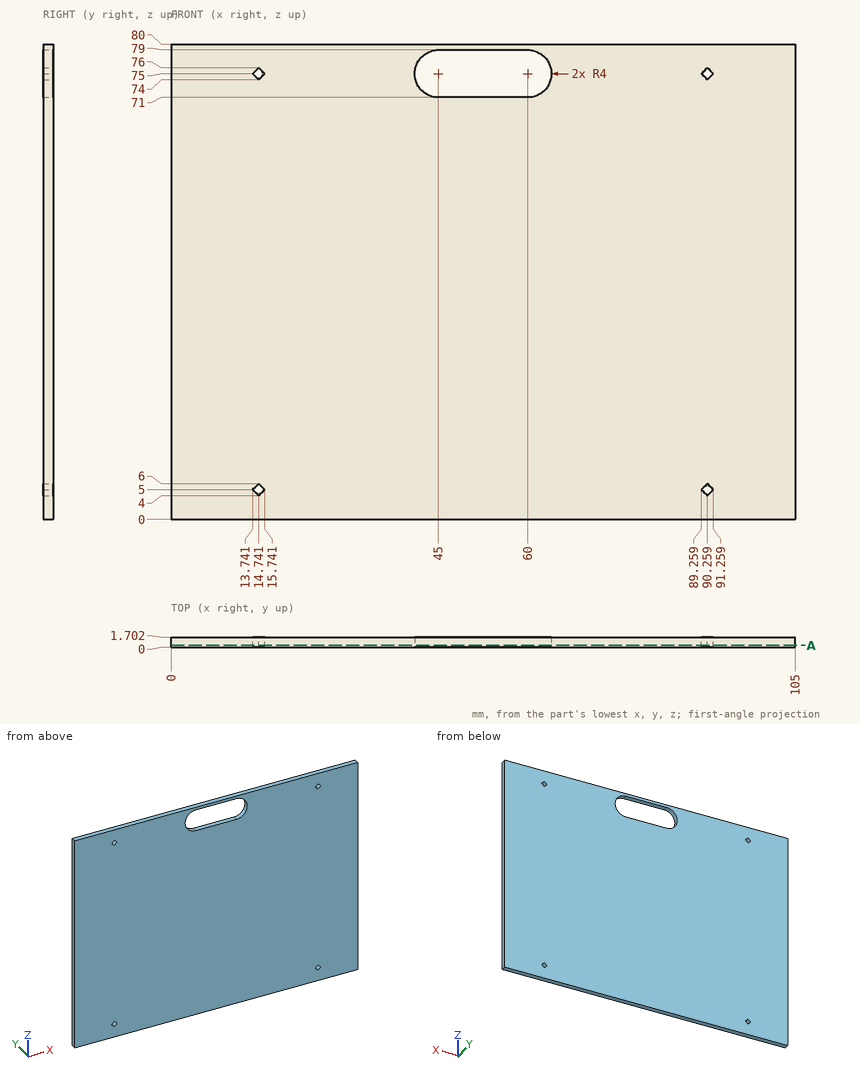
For this review, use the dimensioned drawing (mm, ordinates from the lowest corner) and the shaded views. Coordinates: 2 decimals unless noted, no trailing zeros. Loops run counter-clockwise (first coordinate to the right, second up) from the corner with the lowest first, then second, coordinate; pieces in that order, holes last. Notation, with made-up numbers: (72, 2) -> (100, 2) arc R27 ccw to (100, 26) -> close; hole circle Ø10 at (-17.75, 1). An arc over 180 degrees is marked (long way). Use a Markdown table: item, result. Add a question column.
1. Add section A-A on y = 0.35. Write out the cut boundary in (x, z), plus the area to 3 significant figures.
2. Clearance check with a flat-ended pin moving along its axis: pin 1 Ø4 at (x, z) = (93, 28) entering from -Y. State where the tip first meets the part, or that it passes through.
3. To check wall thickness, follow line 1 (Z direction, x = 91, y = 0.3); line 2 (Z direction, x = 58, y = 1.15); line 3 (X direction, y = 0.8, z = 73) (1 decimal). State the ranges of each line that lie inside material, in increasing order.
Returned:
| question | item | result |
|---|---|---|
| 1 | outline | (0, 0) -> (105, 0) -> (105, 80) -> (0, 80) -> close; hole (13.74, 5) -> (14.74, 4) -> (15.74, 5) -> (14.74, 6) -> close; hole (13.74, 75) -> (14.74, 74) -> (15.74, 75) -> (14.74, 76) -> close; hole (45, 71) -> (60, 71) arc R4 ccw to (60, 79) -> (45, 79) arc R4 ccw to start; hole (89.26, 5) -> (90.26, 4) -> (91.26, 5) -> (90.26, 6) -> close; hole (89.26, 75) -> (90.26, 74) -> (91.26, 75) -> (90.26, 76) -> close |
| 1 | area | 8,220 mm² |
| 2 | pin 1 | stops at y = 0 |
| 3 | line 1 | z = 0 to 4.74, 5.26 to 74.74, 75.26 to 80 |
| 3 | line 2 | z = 0 to 71, 79 to 80 |
| 3 | line 3 | x = 0 to 41.5, 63.5 to 105 |
